Geometry: final body of the model. Coordinates: model frame, mm. A direction names the side the tool comes from. Coordinates: 2 decimals unless noted, no trailing zeros. Loops run counter-clockwise (first coordinate to the right, second up) from the corner with the lowest first, then second, coordinate; pieces in that order, holes last. Notation, with made-up numbers: (88, -8.75) -> (131, -8.75) arc R23 ccw to (131, 8.25) -> close; hole circle Ø5 at (-27.75, -26.5). An arc over 180 degrees is marked (long way). One line per item, written item: value. Start each with the question number.
Item 1: Section query B-B on z = 18. Return loops of the section in (x, y).
Item 2: Section query C-C on x = -3. Return loops of the section in (y, z), then the cut area to 3 significant figures.
Item 3: Ray query, probe 1 along X at (y, z) = (922.75, 16.5); probe 2 along Z at (x, y) = (8, 920); probe 3 along Y at (x, z) = (11, 36.5). Return the intervals inside material, ascending. Write a range as from..to.
Item 4: Section query A-A on y = 922. Return loops of the section in (x, z).
Item 5: Contact query for flat-ended pins moving along their axis: pin 1 Ø1.5 at (x, y) = (-1, 932) entering from -Z; pin 2 Ø3 at (x, z) = (-3, 77) entering from -Y; pin 3 Ø1.5 at (y, z) = (931.5, 33) entering from +X. Output: stop coordinate, or through.
Item 6: Section query D-D on z = 37. Return loops of the section in (x, y), then the cut area to 3 significant figures.
Item 7: Set-up query: faces 5 (the flat face through (0, 933, 38)), 6 (the flat face through (-3, 922, 95)), 7 (the cylindrical face through (20.255, 914.776, 49.767)). Return all of +Z, -Z, +X, -X, +Y, -Y with unobstructed straight access to the full face (end or side cutting, diameter ignored); none if empty.
Item 8: Mould query, pull axis Z, two halves, no side actions, for faces 1 (the flat face through (-20, 922, 51)), 2 (the cylindrical face through (-24, 922, 98)), 3 (the flat face through (0, 935, 49)), 4 (the flat face through (-23, 919.658, 87)). Classes: +Z half, -Z half, draft (parallel to the pull), parting line (faces both ways), or undercut.
from build123d import *

# Parameters (mm, degrees)
BOSS_EXTRUDE1_DEPTH = 100
SKETCH4_W           = 40
SKETCH4_H           = 90
CUT_EXTRUDE1_DEPTH  = 150
SKETCH6_W           = 50
SKETCH6_H           = 100
SKETCH6_W_2         = 15.5
SKETCH6_H_2         = 15.5
BOSS_EXTRUDE2_DEPTH = 5
FILLET1_R           = 5
SKETCH7_W           = 15
SKETCH7_H           = 5
CUT_EXTRUDE2_DEPTH  = 5


with BuildPart() as part:
    # Sketch3 → Boss-Extrude1 (new body)
    with BuildSketch(Plane.XY):
        with BuildLine():
            Line((25, 935), (-25, 935))
            Line((-25, 935), (-25, 914.658406182))
            ThreePointArc((-25, 914.658406182), (0, 915), (25, 914.658406182))
            Line((25, 914.658406182), (25, 935))
        make_face()
    extrude(amount=BOSS_EXTRUDE1_DEPTH)

    # Sketch4 → Cut-Extrude1 (cut)
    with BuildSketch(Plane(origin=(0, 935, 0), x_dir=(1, 0, 0), z_dir=(0, 1, 0))):
        with Locations((0, -50)):
            Rectangle(SKETCH4_W, SKETCH4_H)
    extrude(amount=-CUT_EXTRUDE1_DEPTH, mode=Mode.SUBTRACT)

    # Sketch6 → Boss-Extrude2 (add)
    with BuildSketch(Plane(origin=(0, 935, 0), x_dir=(1, 0, 0), z_dir=(0, 1, 0))):
        with Locations((0, -50)):
            Rectangle(SKETCH6_W, SKETCH6_H)
        with Locations((0, -30.25)):
            Rectangle(SKETCH6_W_2, SKETCH6_H_2, mode=Mode.SUBTRACT)
    extrude(amount=-BOSS_EXTRUDE2_DEPTH)

    # Fillet1
    fillet1_edges = [part.edges().sort_by_distance(p)[0] for p in [
        (25, 924.829203091, 100),
        (0, 935, 100),
        (-25, 924.829203091, 100),
        (-25, 924.829203091, 0),
        (0, 935, 0),
        (25, 924.829203091, 0),
        (-25, 935, 50),
        (25, 935, 50),
    ]]
    fillet(fillet1_edges, radius=FILLET1_R)

    # Sketch7 → Cut-Extrude2 (cut)
    with BuildSketch(Plane.ZY.offset(25)):
        with Locations((87.5, 917.158406182)):
            Rectangle(SKETCH7_W, SKETCH7_H)
    extrude(amount=-CUT_EXTRUDE2_DEPTH, mode=Mode.SUBTRACT)


solid = part.part
Reply:
1. outline: (-25, 914.66) arc R915 cw to (-20, 914.78) -> (-20, 930) -> (20, 930) -> (20, 914.78) arc R915 cw to (25, 914.66) -> (25, 930) arc R5 ccw to (20, 935) -> (-20, 935) arc R5 ccw to (-25, 930) -> close
2. outline: (915, 0) -> (930, 0) arc R5 ccw to (935, 5) -> (935, 22.5) -> (930, 22.5) -> (930, 5) -> (915, 5) -> close; (915, 95) -> (930, 95) -> (930, 38) -> (935, 38) -> (935, 95) arc R5 ccw to (930, 100) -> (915, 100) -> close
2. area: 562 mm²
3. probe 1: x = -25..-20, 20..25
3. probe 2: z = 0..5, 95..100
3. probe 3: y = 930..935
4. outline: (-25, 5) arc R5 ccw to (-20, 0) -> (20, 0) arc R5 ccw to (25, 5) -> (25, 95) arc R5 ccw to (20, 100) -> (-20, 100) arc R5 ccw to (-25, 95) -> close; hole (-20, 5) -> (20, 5) -> (20, 95) -> (-20, 95) -> close
5. pin 1: stops at z = 0.16
5. pin 2: stops at y = 930
5. pin 3: stops at x = 24.94
6. outline: (-25, 914.66) arc R915 cw to (-20, 914.78) -> (-20, 930) -> (-7.75, 930) -> (-7.75, 935) -> (-20, 935) arc R5 ccw to (-25, 930) -> close; (7.75, 930) -> (20, 930) -> (20, 914.78) arc R915 cw to (25, 914.66) -> (25, 930) arc R5 ccw to (20, 935) -> (7.75, 935) -> close
6. area: 315 mm²
7. face 5: +Y, -Y
7. face 6: -Y
7. face 7: +Z, -Z, -Y
8. face 1: undercut
8. face 2: +Z half
8. face 3: draft
8. face 4: undercut
